The listing builds one solid part. Answer for the finished solid, in the listing's coordinates (mm). A direction names the side the tool comes from. Coordinates: 2 decimals unless noted, no trailing zeros. Write each loop counter-clockwise with the first axis right and the second up, starting at its lowest first coordinate (ties: lowest second). Pieces come first, ordered by that corner, then holes.
(1) Which of the six approach directions +Z, -Z, +X, -X, +Y, -Y give full straight-line access (tool end or side, diameter ignored) to faces 1 (the flat face through (0, 25, -20)), 2 (the cylindrical face through (-45.511, 2.465, -53.547)), 3 (the flat face through (-65, 5, -34.5))?
(2) Given P1, Ø12, axis at x = -19, y = 10.5, coming from the -Z side; P2, Ø3, axis at x = -40, y = 30.5, coming from the +Z side; P3, Ø12, axis at y = 9.5, z = -80, coming from the +X side; P4, Ø22, axis at x = -42.5, z = -54, coming from the +Y side, each flat-ended and moving along its own axis, determine where each tip first touches the part or whether it passes through.
(3) For a pull along Y with two mould halves and no side action, classify faces 4 (the cylindrical face through (-55.977, 24.748, -42.801)), 5 (the flat face through (-51, 50, -50)), 6 (the cylindrical face through (-73.48, 2.46, -24.95)) as +Y half, -Y half, draft (parallel to the pull), parting line (faces both ways), or undercut.
(4) Straight lines are drawn through the part: line 1 (Y direction, x = -38, z = -39.5); line 2 (X direction, y = 33.5, z = -88.5); line 3 (Z direction, x = -56.5, y = 36). For each, find the intervals that lie inside material, in ascending order.
(5) The part is cut by section B-B on y = 26. Determine the outline of the cut face in (x, z), plus the area to 3 significant figures.
(6) The part is cut by section A-A on y = 46.5. Determine the outline of the cut face in (x, z), plus the area to 3 significant figures.
Autodesk Inventor part; units mm, degrees
ref_plane "YZ Plane" through (0, 0, 0) normal (1, 0, 0) x (0, 1, 0)
ref_plane "XZ Plane" through (0, 0, 0) normal (0, 1, 0) x (-1, 0, 0)
ref_plane "XY Plane" through (0, 0, 0) normal (0, 0, 1) x (1, 0, 0)
sketch "Sketch1" plane through (0, 0, 0) normal (0, 1, 0) x (-1, 0, 0)
  line L0 (0, 0) -> (141.4214, 0) construction
  line L1 (100, 0) -> (0, 0)
  arc A0 (100.1961, -98.1961) -> (1.8039, 0.1961) centre (10.63, -89.37) ccw
  arc A1 (59.9366, -97.6681) -> (2.3319, -40.0634) centre (10.63, -89.37) ccw
  line L2 (98.2058, -100) -> (61.9088, -100)
  line L3 (0, -1.7942) -> (0, -38.0912)
  arc A2 (98.2058, -100) -> (100.1961, -98.1961) centre (98.2058, -98) ccw
  arc A3 (59.9366, -97.6681) -> (61.9088, -100) centre (61.9088, -98) ccw
  arc A4 (0, -38.0912) -> (2.3319, -40.0634) centre (2, -38.0912) ccw
  arc A5 (1.8039, 0.1961) -> (0, -1.7942) centre (2, -1.7942) ccw
  point P0 (100, -100)
  point P1 (59.4869, -100)
  point P2 (0, -40.5131)
  dimension "d2" = 100
  dimension "d3" = 90
  dimension "d4" = 40
  dimension "d7" = 2
extrude "Extrusion1" add sketch "Sketch1" along normal blind 5
sketch "Sketch2" plane through (0, 5, 0) normal (0, 1, 0) x (1, 0, 0)
  arc A0 (-98.2058, 100) -> (-100.1961, 98.1961) centre (-98.2058, 98) ccw
  arc A1 (-100.1961, 98.1961) -> (-1.8039, -0.1961) centre (-10.63, 89.37) ccw
  arc A2 (-1.8039, -0.1961) -> (0, 1.7942) centre (-2, 1.7942) ccw
  line L0 (0, 1.7942) -> (0, 38.0912)
  arc A3 (0, 38.0912) -> (-2.3319, 40.0634) centre (-2, 38.0912) ccw
  arc A4 (-59.9366, 97.6681) -> (-2.3319, 40.0634) centre (-10.63, 89.37) ccw
  arc A5 (-59.9366, 97.6681) -> (-61.9088, 100) centre (-61.9088, 98) ccw
  line L1 (-61.9088, 100) -> (-98.2058, 100)
  arc A6 (-84.8728, 100) -> (0, 15.1272) centre (-10.63, 89.37) ccw
  arc A7 (-74.7549, 100) -> (0, 25.2451) centre (-10.63, 89.37) ccw
  line L2 (0, 15.1272) -> (0, 25.2451)
  line L3 (-84.8728, 100) -> (-74.7549, 100)
  point P0 (0, 0)
  dimension "d10" = 15
extrude "Extrusion2" add sketch "Sketch2" along normal blind 40 contours L1 A7 L0 A6
fillet "Fillet1" radius 2 2 edges at (-63.663, 5, -36.337) (-56.5919, 5, -43.4081)
sketch "Sketch3" plane through (0, 45, 0) normal (0, 1, 0) x (1, 0, 0)
  arc A0 (-86.8927, 100) -> (0, 13.1073) centre (-10.63, 89.37) ccw
  line L0 (-86.8927, 100) -> (-98.2058, 100)
  arc A1 (-98.2058, 100) -> (-100.1961, 98.1961) centre (-98.2058, 98) ccw
  arc A2 (-100.1961, 98.1961) -> (-1.8039, -0.1961) centre (-10.63, 89.37) ccw
  arc A3 (-1.8039, -0.1961) -> (0, 1.7942) centre (-2, 1.7942) ccw
  line L1 (0, 1.7942) -> (0, 13.1073)
  arc A4 (-72.7267, 100) -> (0, 27.2733) centre (-10.63, 89.37) ccw
  line L2 (0, 27.2733) -> (0, 38.0912)
  arc A5 (0, 38.0912) -> (-2.3319, 40.0634) centre (-2, 38.0912) ccw
  arc A6 (-59.9366, 97.6681) -> (-2.3319, 40.0634) centre (-10.63, 89.37) ccw
  arc A7 (-59.9366, 97.6681) -> (-61.9088, 100) centre (-61.9088, 98) ccw
  line L3 (-61.9088, 100) -> (-72.7267, 100)
  arc A8 (-84.8728, 100) -> (0, 15.1272) centre (-10.63, 89.37) ccw
  line L4 (0, 15.1272) -> (0, 25.2451)
  arc A9 (-74.7549, 100) -> (0, 25.2451) centre (-10.63, 89.37) ccw
  line L5 (-74.7549, 100) -> (-84.8728, 100)
  arc A10 (-74.7549, 100) -> (0, 25.2451) centre (-10.63, 89.37) ccw
  arc A11 (-86.8927, 100) -> (0, 13.1073) centre (-10.63, 89.37) ccw
  line L6 (0, 27.2733) -> (0, 25.2451)
  line L7 (0, 15.1272) -> (0, 13.1073)
  line L8 (-72.7267, 100) -> (-74.7549, 100)
  line L9 (-74.7549, 100) -> (-84.8728, 100)
  line L10 (-86.8927, 100) -> (-84.8728, 100)
  point P0 (0, 0)
extrude "Extrusion3" add sketch "Sketch3" along normal blind 5
fillet "Fillet2" radius 2 2 edges at (-56.5919, 45, -43.4081) (-63.663, 45, -36.337)
properties part number "Curved 100mm"
Model answer:
1. face 1: +Z, -Z, +X, +Y, -Y
1. face 2: +Y, -Y
1. face 3: +Z, -X
2. P1: stops at z = -40.54
2. P2: stops at z = -19.74
2. P3: stops at x = -58.82
2. P4: stops at y = 50
3. face 4: undercut
3. face 5: +Y half
3. face 6: draft
4. line 1: y = 0 to 5, 45 to 50
4. line 2: x = -85.62 to -75.62
4. line 3: z = -43.32 to -30.03
5. outline: (-84.87, -100) - (-74.75, -100) arc R65 cw to (0, -25.25) - (0, -15.13) arc R75 ccw to start
5. area: 1,310 mm2
6. outline: (-100.2, -98.2) arc R2 ccw to (-98.21, -100) - (-61.91, -100) arc R2 ccw to (-59.94, -97.67) arc R50 cw to (-2.33, -40.06) arc R2 ccw to (0, -38.09) - (0, -1.79) arc R2 ccw to (-1.8, 0.2) arc R90 ccw to start
6. area: 5,250 mm2
